Autodesk Inventor part; units mm, degrees
ref_plane "YZ Plane" through (0, 0, 0) normal (1, 0, 0) x (0, 1, 0)
ref_plane "XZ Plane" through (0, 0, 0) normal (0, 1, 0) x (-1, 0, 0)
ref_plane "XY Plane" through (0, 0, 0) normal (0, 0, 1) x (1, 0, 0)
sketch "Sketch1" plane through (0, 0, 0) normal (0, 1, 0) x (-1, 0, 0)
  point P0 (0, 0)
sketch "Sketch2" plane through (0, 0, 0) normal (0, 1, 0) x (-1, 0, 0)
  line L0 (0, 0) -> (33.2, 0)
  line L1 (33.2, 0) -> (33.2, -33.2)
  line L2 (33.2, -33.2) -> (0, -33.2)
  line L3 (0, -33.2) -> (0, 0)
  dimension "d0" = 33.2
  dimension "d1" = 33.2
extrude "Extrusion1" add sketch "Sketch2" along normal blind 2
sketch "Sketch3" plane through (0, 2, 0) normal (0, 1, 0) x (1, 0, 0)
  line L0 (0, 33.2) -> (-33.2, 33.2)
  line L1 (-33.2, 33.2) -> (-33.2, 0)
  line L2 (-33.2, 0) -> (0, 0)
  line L3 (0, 0) -> (0, 33.2)
  line L4 (-33.2, 0) -> (0, 0)
  line L5 (0, 0) -> (-1.2, 0)
  line L6 (-1.2, 0) -> (-1.2, 1.2)
  line L7 (-1.2, 1.2) -> (-32, 1.2)
  line L8 (-32, 1.2) -> (-32, 32)
  line L9 (-32, 32) -> (-1.2, 32)
  line L10 (-1.2, 32) -> (-1.2, 1.2)
  dimension "d4" = 1.2
  dimension "d5" = 1.2
  dimension "d6" = 30.8
  dimension "d7" = 30.8
extrude "Extrusion2" add sketch "Sketch3" along normal blind 4
chamfer "Chamfer1" distance 0.6 angle 45 8 edges at (-1.2, 6, -16.6) (-16.6, 6, -32) (-16.6, 6, -33.2) (0, 6, -16.6) (-16.6, 6, 0) (-16.6, 6, -1.2) (-33.2, 6, -16.6) (-32, 6, -16.6)
sketch "Sketch4" plane through (0, 2, 0) normal (0, 1, 0) x (1, 0, 0)
  line L0 (-1.2, 1.2) -> (-1.2, 32)
  line L1 (-1.2, 32) -> (-32, 32)
  line L2 (-32, 32) -> (-32, 1.2)
  line L3 (-32, 1.2) -> (-1.2, 1.2)
  line L4 (-1.2, 1.2) -> (-1.2, 32)
  line L5 (-1.2, 16.6) -> (-32, 16.6)
  line L6 (-32, 32) -> (-1.2, 32)
  line L7 (-16.6, 32) -> (-16.6, 1.2)
  line L8 (-16.6, 16.6) -> (-16.6, 17.6)
  line L9 (-32, 16.6) -> (-32, 17.6)
  line L10 (-32, 1.2) -> (-32, 32)
  line L11 (-32, 17.6) -> (-30.5, 17.6)
  line L12 (-30.5, 17.6) -> (-30.5, 23.6)
  line L13 (-30.5, 23.6) -> (-32, 23.6)
  line L14 (-30.5, 16.6) -> (-30.5, 15.6)
  line L15 (-30.5, 15.6) -> (-32, 15.6)
  line L16 (-30.5, 15.6) -> (-30.5, 9.6)
  line L17 (-30.5, 9.6) -> (-32, 9.6)
  line L18 (-1.2, 16.6) -> (-1.2, 17.6)
  line L19 (-1.2, 17.6) -> (-2.7, 17.6)
  line L20 (-2.7, 17.6) -> (-2.7, 23.6)
  line L21 (-2.7, 23.6) -> (-1.2, 23.6)
  line L22 (-1.2, 16.6) -> (-1.2, 15.6)
  line L23 (-1.2, 15.6) -> (-2.7, 15.6)
  line L24 (-2.7, 9.6) -> (-2.7, 15.6)
  line L25 (-2.7, 9.6) -> (-1.2, 9.6)
  point P0 (0, 0)
  dimension "d13" = 1
  dimension "d14" = 1.5
  dimension "d15" = 6
  dimension "d16" = 1
  dimension "d17" = 6
  dimension "d18" = 1
  dimension "d19" = 1.5
  dimension "d20" = 6
extrude "Extrusion3" cut sketch "Sketch4" against normal blind 4 contours L25 L24 L23 L0 | L2 L15 L16 L17 | L19 L20 L21 L0 | L2 L13 L12 L11
sketch "Sketch5" plane through (0, 0, 0) normal (0, -1, 0) x (1, 0, 0)
  line L0 (-1.2, -17.6) -> (-1.2, -23.6)
  line L1 (-1.2, -23.6) -> (-2.7, -23.6)
  line L2 (-2.7, -23.6) -> (-2.7, -17.6)
  line L3 (-2.7, -17.6) -> (-1.2, -17.6)
  line L4 (-32, -23.6) -> (-32, -17.6)
  line L5 (-32, -17.6) -> (-30.5, -17.6)
  line L6 (-30.5, -17.6) -> (-30.5, -23.6)
  line L7 (-30.5, -23.6) -> (-32, -23.6)
  line L8 (-1.2, -9.6) -> (-1.2, -15.6)
  line L9 (-1.2, -15.6) -> (-2.7, -15.6)
  line L10 (-2.7, -15.6) -> (-2.7, -9.6)
  line L11 (-2.7, -9.6) -> (-1.2, -9.6)
  line L12 (-32, -15.6) -> (-32, -9.6)
  line L13 (-32, -9.6) -> (-30.5, -9.6)
  line L14 (-30.5, -9.6) -> (-30.5, -15.6)
  line L15 (-30.5, -15.6) -> (-32, -15.6)
  line L16 (0, -33.2) -> (-33.2, -33.2)
  line L17 (0, 0) -> (0, -33.2)
  line L18 (-33.2, 0) -> (0, 0)
  line L19 (-33.2, -33.2) -> (-33.2, 0)
  line L20 (-33.2, 0) -> (0, 0)
  line L21 (-16.6, 0) -> (-16.6, -33.2)
  line L22 (0, -33.2) -> (-33.2, -33.2)
  line L23 (-16.6, -16.6) -> (-16.6, -1.6)
  line L24 (-1.2, -1.2) -> (-32, -1.2)
  line L25 (-16.6, -1.6) -> (-10.1, -1.6)
  line L26 (-10.1, -1.6) -> (-10.1, -31.6)
  line L27 (-10.1, -31.6) -> (-23.1, -31.6)
  line L28 (-23.1, -31.6) -> (-23.1, -1.6)
  line L29 (-23.1, -1.6) -> (-16.6, -1.6)
  line L30 (-10.1, -1.6) -> (-11.1, -1.6)
  line L31 (-11.1, -1.6) -> (-11.1, -2.6)
  line L32 (-11.1, -2.6) -> (-22.1, -2.6)
  line L33 (-22.1, -2.6) -> (-22.1, -30.6)
  line L34 (-22.1, -30.6) -> (-11.1, -30.6)
  line L35 (-11.1, -30.6) -> (-11.1, -2.6)
  dimension "d25" = 6.5
  dimension "d26" = 30
  dimension "d27" = 13
  dimension "d28" = 1
  dimension "d29" = 1
  dimension "d30" = 11
  dimension "d31" = 28
extrude "Extrusion4" cut sketch "Sketch5" against normal blind 1 contours L27 L28 L29 L21 L32 L33 L34 | L21 L34 L35 L31 L25 L26 L27 | L25 L31 L32 L21
chamfer "Chamfer2" distance 0.5 angle 45 8 edges at (-11.1, 1, -16.6) (-16.6, 1, -2.6) (-23.1, 1, -16.6) (-16.6, 1, -1.6) (-22.1, 1, -16.6) (-10.1, 1, -16.6) (-16.6, 1, -30.6) (-16.6, 1, -31.6)
properties part number "led-compartment"
Can you work these out from the model? Positions are in its coordinate system, mm. A direction names the side the tool comes from. Coordinates: 2 decimals unless noted, no trailing zeros. Order: outer loops, then holes, each group sorted by start corner. A loop starts at its lowest first (then second) coordinate and runs counter-clockwise, first axis right, second up. Notation, with made-up numbers: M 57.5,-17.75 L 102.5,-17.75 A38 cw 102.5,20.25 Z; hole C -40,59 d3. An arc over 180 degrees is marked long. Write item = value, one per line.
(1) If we mould it in two halves opening along Z, with no side actions, what happens to faces 1 (the face through (-16, 4, -1.2)), 2 (the face through (-16, 3, 0)), 3 (the face through (0, 3, -17))? For each: pulls with the +Z half, pulls with the -Z half, needs draft (parallel to the pull), parting line crosses it, or undercut.
Results are:
face_1 = undercut
face_2 = pulls with the +Z half
face_3 = needs draft
(2) For pin 1 Ø1.5 at (x, z) = (-20, -7.5) entering from +Y, with a flat end and sliding along its axis, tell me the tip position at first contact or that it passes through.
Results are:
pin_1 = 2
(3) For faces 4 (the face through (-2.7, 1, -13)), 5 (the face through (-33.2, 3, -16)), 6 (the face through (-16, 2, -16)), which set-ups out of +Z, -Z, +X, -X, +Y, -Y let a thin tool reach every point of the face, with its end or its side?
Results are:
face_4 = +Y, -Y
face_5 = +Z, -Z, -X, +Y, -Y
face_6 = +Y
(4) Suppose I cut it at B-B on y = 5. Please give me the cut outline in (x, z).
Results are:
outline = M -33.2,-33.2 L 0,-33.2 L 0,0 L -33.2,0 Z; hole M -32,-32 L -1.2,-32 L -1.2,-1.2 L -32,-1.2 Z
(5) I need wall thicknesses on line 1 along X through (y, z) = (0.5, -3); line 2 along X through (y, z) = (4.75, -28.5). Which ranges of each line are inside material? Lowest first, please. Write a range as [from, to].
Results are:
line_1 = [-33.2, -23.1], [-22.1, -11.1], [-10.1, 0]
line_2 = [-33.2, -32], [-1.2, 0]
